```python
from build123d import *

# Parameters (mm, degrees)
SKETCH1_W           = 50
SKETCH1_H           = 105
BOSS_EXTRUDE1_DEPTH = 9
SKETCH2_R           = 11
SKETCH2_R_2         = 1.85
SKETCH2_R_3         = 5.1
CUT_EXTRUDE1_DEPTH  = 9
SKETCH3_R           = 1.85
CUT_EXTRUDE4_DEPTH  = 10
FILLET1_R           = 15


with BuildPart() as part:
    # Sketch1 → Boss-Extrude1 (new body)
    with BuildSketch(Plane(origin=(0, 0, 0), x_dir=(1, 0, 0), z_dir=(0, 1, 0))):
        with Locations((34.488967371, 40.084311239)):
            Rectangle(SKETCH1_W, SKETCH1_H)
    extrude(amount=BOSS_EXTRUDE1_DEPTH)

    # Sketch2 → Cut-Extrude1 (cut)
    with BuildSketch(Plane(origin=(0, 9, 0), x_dir=(1, 0, 0), z_dir=(0, 1, 0))):
        with Locations((34.488967371, 7.584311239)):
            Circle(SKETCH2_R)
        with Locations((49.988967371, 23.084311239)):
            Circle(SKETCH2_R_2)
        with Locations((18.988967371, -7.915688761)):
            Circle(SKETCH2_R_2)
        with Locations((49.988967371, -7.915688761)):
            Circle(SKETCH2_R_2)
        with Locations((18.988967371, 23.084311239)):
            Circle(SKETCH2_R_2)
        with Locations((52.488967371, 82.584311239)):
            Circle(SKETCH2_R_2)
        with Locations((34.488967371, 82.584311239)):
            Circle(SKETCH2_R_3)
        with Locations((16.488967371, 82.584311239)):
            Circle(SKETCH2_R_2)
        with BuildLine():
            Line((21.488967371, 50.984311239), (11.488967371, 50.984311239))
            ThreePointArc((11.488967371, 50.984311239), (9.888967371, 52.584311239), (11.488967371, 54.184311239))
            Line((11.488967371, 54.184311239), (21.488967371, 54.184311239))
            ThreePointArc((21.488967371, 54.184311239), (23.088967371, 52.584311239), (21.488967371, 50.984311239))
        make_face()
    extrude(amount=-CUT_EXTRUDE1_DEPTH, mode=Mode.SUBTRACT)

    # Sketch3 → Cut-Extrude4 (cut)
    with BuildSketch(Plane(origin=(0, 9, 0), x_dir=(1, 0, 0), z_dir=(0, 1, 0))):
        with Locations((14.488967371, 40.584311239)):
            Circle(SKETCH3_R)
        with Locations((54.488967371, 40.584311239)):
            Circle(SKETCH3_R)
        with Locations((54.488967371, 33.084311239)):
            Circle(SKETCH3_R)
        with Locations((14.488967371, 33.084311239)):
            Circle(SKETCH3_R)
    extrude(amount=-CUT_EXTRUDE4_DEPTH, mode=Mode.SUBTRACT)

    # Fillet1
    fillet1_edges = [part.edges().sort_by_distance(p)[0] for p in [
        (9.488967371, 4.5, -92.584311239),
        (59.488967371, 4.5, -92.584311239),
        (59.488967371, 4.5, 12.415688761),
        (9.488967371, 4.5, 12.415688761),
    ]]
    fillet(fillet1_edges, radius=FILLET1_R)


solid = part.part
```
Can you work these out from the model? Positions are in its coordinate system, mm. A direction names the side the tool comes from. Round coordinates to 2 decimals unless told otherwise and drop trailing zeros. Loops run counter-clockwise (first coordinate to the right, second up) from the corner with the lowest first, then second, coordinate; pieces in that order, holes last. Notation, with made-up numbers: M 52,86 L 107,86 A15 ccw 107,112 Z; hole C 15,27 d10. An arc over 180 degrees is marked long. Write item = value, one per line. Start each with the question number.
(1) Suppose I cut it at B-B on y = 3.25. Give the number of separate pieces and of enclosed holes in the cut face, plus the area to 3 significant figures.
(2) I need wall thicknesses on line 1 along Z through (x, y) = (55, 6.5); line 2 along Z through (x, y) = (31.5, 6); line 3 along X through (y, z) = (1.75, -3). Which ranges of each line are inside material? Lowest first, please.
(3) Suppose I cut it at A-A on x = 36. Write out the boundary of the cut face in (y, z).
(4) I'm going to push flat-ended pins straight in: P1, Ø4, axis at y = 3.5, z = -82, coming from the +X side; P2, Ø4.5, axis at x = 49.99, z = -23.08, coming from the -Y side; P3, Ø20, axis at x = 34.49, z = -7.58, coming from the +Y side. Where does each tip first touch, or does it pass through?
(5) Which directions (+Z, -Z, +X, -X, +Y, -Y) give clear straight access to the entire face, cutting with the end or side of a thin tool? Please do faces 5 (the face through (17, 5, -50.984)), 6 (the face through (34, 4, 12.416)).
(6) If we mould it in two halves opening along X, with no side actions, what happens to faces 1 (the face through (54.978, 4.563, -88.307)), 2 (the face through (15.34, 4.56, -31.44)), 3 (the face through (34, 4, -92.584)), 4 (the face through (13.766, 4.563, -88.074))? For each: released by +X, released by -X, zero draft, split by the parting line, or undercut.
Answer block:
q1.separate_pieces = 1
q1.enclosed_holes = 13
q1.area = 4,450 mm²
q2.line_1 = -88.29 to -42.36, -38.81 to -34.86, -31.31 to 8.12
q2.line_2 = -92.58 to -86.72, -78.45 to -18.17, 3 to 12.42
q2.line_3 = 9.49 to 24.49, 44.49 to 59.49
q3.outline = M 0,-92.58 L 9,-92.58 L 9,-87.46 L 0,-87.46 Z; M 0,-77.71 L 9,-77.71 L 9,-18.48 L 0,-18.48 Z; M 0,3.31 L 9,3.31 L 9,12.42 L 0,12.42 Z
q4.P1 = 59.29
q4.P2 = 0
q4.P3 = through
q5.face_5 = +Y, -Y
q5.face_6 = +Z, +X, -X, +Y, -Y
q6.face_1 = released by +X
q6.face_2 = undercut
q6.face_3 = zero draft
q6.face_4 = released by -X
